```python
from build123d import *

# Parameters (mm, degrees)
SKETCH_1_R          = 2.5
SKETCH_1_R_2        = 5.03
SKETCH_1_R_3        = 2
SKETCH_1_R_4        = 9.53
EXTRUDE_1_DEPTH     = 4
SKETCH_3_W          = 46.2
SKETCH_3_H          = 3.817212264
EXTRUDE_2_DEPTH     = 4
SKETCH_2_R          = 2
SKETCH_2_R_2        = 1.5
SKETCH_2_W          = 32.809844138
SKETCH_2_H          = 42
SKETCH_2_W_2        = 8.2
SKETCH_2_H_2        = 4.2
CUT_EXTRUDE_1_DEPTH = 4


with BuildPart() as part:
    # 草图1 → 凸台-拉伸1 (new body)
    with BuildSketch(Plane.XY):
        with BuildLine():
            ThreePointArc((-1.457142857, 39.854285714), (-41.457142857, -0.145714286), (-1.457142857, -40.145714286))
            Line((-1.457142857, -40.145714286), (328.542857143, -40.145714286))
            ThreePointArc((328.542857143, -40.145714286), (368.542857143, -0.145714286), (328.542857143, 39.854285714))
            Line((328.542857143, 39.854285714), (-1.457142857, 39.854285714))
        make_face()
        with Locations((-1.457142857, -23.895714286)):
            Circle(SKETCH_1_R, mode=Mode.SUBTRACT)
        with Locations((-20.942714442, -11.395714286)):
            Circle(SKETCH_1_R, mode=Mode.SUBTRACT)
        with Locations((18.028428728, -11.395714286)):
            Circle(SKETCH_1_R, mode=Mode.SUBTRACT)
        with Locations((-1.457142857, -0.145714286)):
            Circle(SKETCH_1_R_2, mode=Mode.SUBTRACT)
        with Locations((238.542857143, -16.645714286)):
            Circle(SKETCH_1_R_3, mode=Mode.SUBTRACT)
        with Locations((288.542857143, -0.145714286)):
            Circle(SKETCH_1_R_3, mode=Mode.SUBTRACT)
        with Locations((328.542857143, -0.145714286)):
            Circle(SKETCH_1_R_4, mode=Mode.SUBTRACT)
        with Locations((-22.025246197, 11.729285714)):
            Circle(SKETCH_1_R, mode=Mode.SUBTRACT)
        with Locations((19.110960483, 11.729285714)):
            Circle(SKETCH_1_R, mode=Mode.SUBTRACT)
        with Locations((-1.457142857, 22.354285714)):
            Circle(SKETCH_1_R, mode=Mode.SUBTRACT)
        with Locations((238.542857143, 16.354285714)):
            Circle(SKETCH_1_R_3, mode=Mode.SUBTRACT)
    extrude(amount=EXTRUDE_1_DEPTH)

    # 草图3 → 凸台-拉伸2 (add)
    with BuildSketch(Plane.XY.offset(4)):
        with Locations((18.542857143, -41.36131722)):
            Rectangle(SKETCH_3_W, SKETCH_3_H)
    extrude(amount=-EXTRUDE_2_DEPTH)

    # 草图2 → 切除-拉伸1 (cut)
    with BuildSketch(Plane.XY.offset(4)):
        with Locations((18.542857143, 33.854285714)):
            Circle(SKETCH_2_R)
        with Locations((108.542857143, 33.854285714)):
            Circle(SKETCH_2_R)
        with Locations((198.542857143, 33.854285714)):
            Circle(SKETCH_2_R)
        with Locations((288.542857143, 33.854285714)):
            Circle(SKETCH_2_R)
        with Locations((108.542857143, -34.145714286)):
            Circle(SKETCH_2_R)
        with Locations((198.542857143, -34.145714286)):
            Circle(SKETCH_2_R)
        with Locations((288.542857143, -34.145714286)):
            Circle(SKETCH_2_R)
        with Locations((18.542857143, -40.329923352)):
            Circle(SKETCH_2_R_2)
        Polygon((31.542857143, -21.145714286), (104.183898028, -21.145714286), (159.772133322, 20.854285714), (31.542857143, 20.854285714), align=None)
        Polygon((148.123425102, -21.145714286), (203.711660396, 20.854285714), (233.542857143, 20.854285714), (233.542857143, -21.145714286), align=None)
        with Locations((259.947779212, -0.145714286)):
            Rectangle(SKETCH_2_W, SKETCH_2_H)
        with Locations((33.542857143, -40.329923352)):
            Rectangle(SKETCH_2_W_2, SKETCH_2_H_2)
        with Locations((3.542857143, -40.329923352)):
            Rectangle(SKETCH_2_W_2, SKETCH_2_H_2)
    extrude(amount=-CUT_EXTRUDE_1_DEPTH, mode=Mode.SUBTRACT)


solid = part.part
```
Geometry: final body of the model. Coordinates: model frame, mm. A direction names the side the tool comes from. Give positions to 0.01 mm unless a question says otherwise; leave off trailing zeros. Loops run counter-clockwise (first coordinate to the right, second up) from the corner with the lowest first, then second, coordinate; pieces in that order, holes last. Notation, with made-up numbers: (67.5, 87.5) - (91.5, 87.5) arc R14 ccw to (91.5, 101.5) - close; hole circle Ø8 at (-7.5, 7.25). An arc over 180 degrees is marked (long way). Answer as CSV lines item,"result". Start each with the question number.
(1) Ray query, line 1 along X through (y, z) = (-21, 3.3); line 2 along Y through (x, z) = (77.5, 2.8); line 3 along X through (y, z) = (-14.5, 0.4). Return the intervals inside material, ascending. Write a range as [from, to].
(2) Section query A-A (x = 94). Output: boundary loops of the cut face in (y, z), and give its area (3 significant figures).
(3) Pin query (flat end, axial travel): P1, Ø2, axis at y = -34, z = 2.5, coming from the -X side; P2, Ø1, axis at y = -30, z = 3, coming from the +X side (3 decimals); P3, Ø3.5, axis at x = 288.54, y = 33.85, coming from the -Z side; P4, Ø2, axis at y = 2.5, z = 3.5, coming from the +X side. Return the tip coordinate at first contact, or that it passes through.
(4) Reachability of faces 1 (the face through (175.53, -0.44, 2.03)), 2 (the face through (161, -1, 4)) from +Z, -Z, +X, -X, +Y, -Y: full face, straight path, thin tool, end or side. Return the list, or none.
(5) Mould query, pull axis Y, two halves, no side actions, for faces 3 (the face through (131.59, -0.44, 2.03)), 4 (the face through (368.533, -1.025, 1.972)), 5 (the face through (161, -1, 0)). Classes: +Y half, -Y half, draft (parallel to the pull), parting line (faces both ways), or undercut.
(6) Section query B-B (z = 2.15). Give the number of separate pieces and of enclosed holes in the cut face, and give its area (3 significant figures).
Worked answers:
1,line 1,"x = [-35.59, 31.54], [104.38, 148.32], [233.54, 243.54], [276.35, 362.68]"
1,line 2,"y = [-40.15, -21.15], [20.85, 39.85]"
1,line 3,"x = [-38.79, 31.54], [112.98, 156.92], [233.54, 243.54], [276.35, 365.88]"
2,outline,"(-40.15, 0) - (-21.15, 0) - (-21.15, 4) - (-40.15, 4) - close; (20.85, 0) - (39.85, 0) - (39.85, 4) - (20.85, 4) - close"
2,area,"152 mm^2"
3,P1,"stops at x = -24.27"
3,P2,"stops at x = 355.715"
3,P3,"passes through"
3,P4,"stops at x = 368.51"
4,face 1,"+Z, -Z"
4,face 2,"+Z, +X, -X, +Y, -Y"
5,face 3,"undercut"
5,face 4,"parting line"
5,face 5,"draft"
6,separate pieces,"1"
6,enclosed holes,"24"
6,area,"22,900 mm^2"
